Autodesk Inventor part; units mm, degrees
ref_plane "YZ Plane" through (0, 0, 0) normal (1, 0, 0) x (0, 1, 0)
ref_plane "XZ Plane" through (0, 0, 0) normal (0, 1, 0) x (-1, 0, 0)
ref_plane "XY Plane" through (0, 0, 0) normal (0, 0, 1) x (1, 0, 0)
sketch "Sketch1" plane through (0, 0, 0) normal (0, 1, 0) x (-1, 0, 0)
  line L0 (0, 0) -> (21.5, 0)
  line L1 (21.5, 0) -> (21.5, -51.5)
  line L2 (21.5, -51.5) -> (0, -51.5)
  line L3 (0, -51.5) -> (0, 0)
  line L4 (23.5, 2) -> (-2, 2)
  line L5 (-2, 2) -> (-2, -53.5)
  line L6 (-2, -53.5) -> (23.5, -53.5)
  line L7 (23.5, -53.5) -> (23.5, 2)
  line L8 (10.75, 0) -> (10.75, -51.5) construction
  circle A0 centre (10.75, -3) radius 1.5
  line L9 (0, -3) -> (21.5, -3) construction
  circle A1 centre (14.75, -3) radius 1.5
  circle A2 centre (18.75, -3) radius 1.5
  circle A3 centre (6.75, -3) radius 1.5
  circle A4 centre (2.75, -3) radius 1.5
  circle A5 centre (18.75, -7) radius 1.5
  circle A6 centre (14.75, -7) radius 1.5
  circle A7 centre (10.75, -7) radius 1.5
  circle A8 centre (6.75, -7) radius 1.5
  circle A9 centre (2.75, -7) radius 1.5
  circle A10 centre (18.75, -11) radius 1.5
  circle A11 centre (14.75, -11) radius 1.5
  circle A12 centre (10.75, -11) radius 1.5
  circle A13 centre (6.75, -11) radius 1.5
  circle A14 centre (2.75, -11) radius 1.5
  circle A15 centre (18.75, -15) radius 1.5
  circle A16 centre (14.75, -15) radius 1.5
  circle A17 centre (10.75, -15) radius 1.5
  circle A18 centre (6.75, -15) radius 1.5
  circle A19 centre (2.75, -15) radius 1.5
  point P0 (10.75, -3)
  point P1 (10.75, -7)
  point P2 (10.75, -11)
  point P3 (10.75, -15)
  dimension "d0" = 21.5
  dimension "d1" = 51.5
  dimension "d2" = 2
  dimension "d3" = 2
  dimension "d4" = 2
  dimension "d5" = 2
  dimension "d6" = 3
  dimension "d8" = 3
  dimension "d9" = 3
  dimension "d10" = 3
  dimension "d11" = 3
  dimension "d12" = 3
  dimension "d13" = 4
  dimension "d14" = 4
  dimension "d15" = 4
  dimension "d16" = 4
  dimension "d19" = 4
extrude "Extrusion1" add sketch "Sketch1" along normal blind 3 contours L0 L1 L2 L3 | L7 L6 L5 L4
fillet "Fillet1" radius 2 8 edges at (-23.5, 3, -25.75) (-10.75, 3, 2) (-23.5, 1.5, 2) (2, 1.5, 2) (2, 3, -25.75) (-10.75, 3, -53.5) (-23.5, 1.5, -53.5) (2, 1.5, -53.5)
sketch "Sketch2" plane through (0, 3, 0) normal (0, 1, 0) x (1, 0, 0)
  line L0 (-17.4247, 49.4836) -> (-8.1758, 49.4836) construction
  line L1 (-8.1758, 49.4836) -> (-8.1758, 43.1661) construction
  line L2 (-8.1758, 43.1661) -> (-17.4247, 43.1661) construction
  line L3 (-17.4247, 43.1661) -> (-17.4247, 49.4836) construction
  spline S0 degree 2 poles (-13.624, 39.127) (-14.7099, 39.127) (-16.2334, 39.5808) (-16.906, 39.905) knots 0 0 0 1 2 2 2
  line L4 (-16.906, 39.905) -> (-16.906, 41.5744)
  line L5 (-16.906, 41.5744) -> (-16.8088, 41.5744)
  spline S1 degree 2 poles (-16.8088, 41.5744) (-16.1524, 40.9585) (-14.4911, 40.2778) (-13.7213, 40.2778) knots 0 0 0 1 2 2 2
  spline S2 degree 2 poles (-13.7213, 40.2778) (-12.6192, 40.2778) (-11.4928, 41.1935) (-11.4928, 41.9471) knots 0 0 0 1 2 2 2
  spline S3 degree 2 poles (-11.4928, 41.9471) (-11.4928, 42.5468) (-12.0843, 43.2923) (-12.7245, 43.4787) knots 0 0 0 1 2 2 2
  spline S4 degree 2 poles (-12.7245, 43.4787) (-13.1864, 43.6084) (-13.9563, 43.7867) (-14.5317, 43.9325) knots 0 0 0 1 2 2 2
  spline S5 degree 2 poles (-14.5317, 43.9325) (-15.0503, 44.0703) (-15.8688, 44.4836) (-16.1848, 44.8158) knots 0 0 0 1 2 2 2
  spline S6 degree 2 poles (-16.1848, 44.8158) (-16.4928, 45.1481) (-16.8331, 46.0395) (-16.8331, 46.623) knots 0 0 0 1 2 2 2
  spline S7 degree 2 poles (-16.8331, 46.623) (-16.8331, 47.8385) (-14.9368, 49.4836) (-13.4701, 49.4836) knots 0 0 0 1 2 2 2
  spline S8 degree 2 poles (-13.4701, 49.4836) (-12.6273, 49.4836) (-11.1362, 49.1513) (-10.496, 48.8353) knots 0 0 0 1 2 2 2
  line L6 (-10.496, 48.8353) -> (-10.496, 47.247)
  line L7 (-10.496, 47.247) -> (-10.5932, 47.247)
  spline S9 degree 2 poles (-10.5932, 47.247) (-11.0714, 47.6846) (-12.5624, 48.3329) (-13.3809, 48.3329) knots 0 0 0 1 2 2 2
  spline S10 degree 2 poles (-13.3809, 48.3329) (-14.3047, 48.3329) (-15.4474, 47.4658) (-15.4474, 46.7607) knots 0 0 0 1 2 2 2
  spline S11 degree 2 poles (-15.4474, 46.7607) (-15.4474, 46.1287) (-14.7748, 45.375) (-14.1427, 45.2048) knots 0 0 0 1 2 2 2
  spline S12 degree 2 poles (-14.1427, 45.2048) (-13.7213, 45.0914) (-12.4976, 44.7996) (-12.0924, 44.6781) knots 0 0 0 1 2 2 2
  spline S13 degree 2 poles (-12.0924, 44.6781) (-11.0633, 44.362) (-10.107, 43.0898) (-10.107, 42.1578) knots 0 0 0 1 2 2 2
  spline S14 degree 2 poles (-10.107, 42.1578) (-10.107, 41.5663) (-10.5851, 40.4317) (-11.0146, 40.0346) knots 0 0 0 1 2 2 2
  spline S15 degree 2 poles (-11.0146, 40.0346) (-11.4928, 39.597) (-12.7083, 39.127) (-13.624, 39.127) knots 0 0 0 1 2 2 2
  line L8 (-3.3728, 39.3053) -> (-8.2513, 39.3053)
  line L9 (-8.2513, 39.3053) -> (-8.2513, 40.3264)
  line L10 (-8.2513, 40.3264) -> (-6.436, 40.3264)
  line L11 (-6.436, 40.3264) -> (-6.436, 47.0282)
  line L12 (-6.436, 47.0282) -> (-8.2513, 47.0282)
  line L13 (-8.2513, 47.0282) -> (-8.2513, 47.9439)
  spline S16 degree 2 poles (-8.2513, 47.9439) (-7.2221, 47.9439) (-6.2496, 48.5274) (-6.1848, 49.3377) knots 0 0 0 1 2 2 2
  line L14 (-6.1848, 49.3377) -> (-5.1475, 49.3377)
  line L15 (-5.1475, 49.3377) -> (-5.1475, 40.3264)
  line L16 (-5.1475, 40.3264) -> (-3.3728, 40.3264)
  line L17 (-3.3728, 40.3264) -> (-3.3728, 39.3053)
  point P0 (0, 0)
extrude "Extrusion2" add sketch "Sketch2" along normal blind 0.5
equation "\"d8\" = d6"
equation "\"d9\" = d11"
equation "\"d10\" = d11"
equation "\"d11\" = d6"
equation "\"d12\" = d11"
equation "\"d14\" = d13"
equation "\"d16\" = d15"
properties part number "sensor1"
Model file for the job. Use its own axes, mm. Give positions to 0.01 mm unless a question says otherwise; leave off trailing zeros. Order: outer loops, then holes, each group sorted by start corner. A loop starts at its lowest first (then second) coordinate and runs counter-clockwise, first axis right, second up.
1) Saw through at A-A, the plane x = -18.75. Write the cut outline in (y, z).
2) Saw through at B-B, the plane z = -7. Write the cut outline in (x, y), then the cut area to 3 significant figures.
3) Mould opens along Z. For faces 1 (the cylindrical face through (-10.9, 2.43, -52.9)), 2 (the cylindrical face through (-10.6, 2.43, 1.4)), 3 (the flat face through (-14, 3.5, -44)), 4 (the cylindrical face through (-1.64, 1.48, -16.01)) say: +Z half, -Z half, draft (parallel to the pull), parting line (faces both ways), or undercut.
4) Wall check: probe 1 along Z at (x, y) = (-14.75, 1); probe 2 along X at (y, z) = (0.5, -2); probe 3 along Z at (x, y) = (-15.25, 1.3). Give the ranges that are in metal, low to high.
5) Saw through at C-C, the plane x = -0.5. Write the cut outline in (y, z), then the cut area to 3 significant figures.
6) Saw through at D-D, the plane y = 2.35. Count the separate pieces of the cut face and the enclosed holes in it, then the cut area to 3 significant figures.
7) Pin check, flat tips, straight feed: pin 1 (1.8 mm diameter, centred on x = -6.75, z = -15, fed in from +Y); pin 2 (4 mm diameter, centred on x = -18.75, z = -3, fed in from +Y); pin 3 (0.6 mm diameter, centred on x = -6, y = 3, fed in from -Z). Stop position of each tip, or through.
Computed:
1. outline: (0, -53.5) - (1, -53.5) arc R2 ccw to (3, -51.5) - (3, -16.5) - (0, -16.5) - close; (0, -13.5) - (3, -13.5) - (3, -12.5) - (0, -12.5) - close; (0, -9.5) - (3, -9.5) - (3, -8.5) - (0, -8.5) - close; (0, -5.5) - (3, -5.5) - (3, -4.5) - (0, -4.5) - close; (0, -1.5) - (3, -1.5) - (3, 0) arc R2 ccw to (1, 2) - (0, 2) - close
2. outline: (-23.5, 0) - (-20.25, 0) - (-20.25, 3) - (-21.5, 3) arc R2 ccw to (-23.5, 1) - close; (-17.25, 0) - (-16.25, 0) - (-16.25, 3) - (-17.25, 3) - close; (-13.25, 0) - (-12.25, 0) - (-12.25, 3) - (-13.25, 3) - close; (-9.25, 0) - (-8.25, 0) - (-8.25, 3) - (-9.25, 3) - close; (-5.25, 0) - (-4.25, 0) - (-4.25, 3) - (-5.25, 3) - close; (-1.25, 0) - (2, 0) - (2, 1) arc R2 ccw to (0, 3) - (-1.25, 3) - close
2. area: 29.8 mm2
3. face 1: -Z half
3. face 2: +Z half
3. face 3: draft
3. face 4: undercut
4. probe 1: z = -53.5 to -16.5, -13.5 to -12.5, -9.5 to -8.5, -5.5 to -4.5, -1.5 to 2
4. probe 2: x = -23.5 to -19.87, -17.63 to -15.87, -13.63 to -11.87, -9.63 to -7.87, -5.63 to -3.87, -1.63 to 2
4. probe 3: z = -53.48 to -16.41, -13.59 to -12.41, -9.59 to -8.41, -5.59 to -4.41, -1.59 to 1.98
5. outline: (0, -53.5) - (1, -53.5) arc R2 ccw to (3, -51.5) - (3, 0) arc R2 ccw to (1, 2) - (0, 2) - close
5. area: 165 mm2
6. separate pieces: 1
6. enclosed holes: 20
6. area: 1,190 mm2
7. pin 1: passes through
7. pin 2: stops at y = 3
7. pin 3: stops at z = -52.55
